from build123d import *

# Parameters (mm, degrees)
SKETCH2_W               = 1.1684
SKETCH2_H               = 0.7874
CUT_EXTRUDE1_DEPTH      = 3.7432
CUT_EXTRUDE1_DEPTH_BACK = 3.7432


with BuildPart() as part:
    # Sketch1 → Revolve1 (revolve)
    with BuildSketch(Plane.XY):
        with BuildLine():
            Line((0, 0), (0, 19.05))
            ThreePointArc((0, 19.05), (1.348059913, 18.449540529), (1.8034, 17.045801767))
            Line((1.8034, 17.045801767), (1.8034, 9.525))
            Line((1.8034, 9.525), (2.7432, 9.525))
            Line((2.7432, 9.525), (2.7432, 0))
            Line((2.7432, 0), (0, 0))
        make_face()
    revolve(axis=Axis((0, 0, 0), (0, 1, 0)))

    # Sketch2 → Cut-Extrude1 (cut, two sides)
    with BuildSketch(Plane.XY) as cut_extrude1_sk:
        with Locations((0, 0.3937)):
            Rectangle(SKETCH2_W, SKETCH2_H)
    extrude(amount=CUT_EXTRUDE1_DEPTH, mode=Mode.SUBTRACT)
    extrude(cut_extrude1_sk.sketch, amount=-CUT_EXTRUDE1_DEPTH_BACK, mode=Mode.SUBTRACT)


solid = part.part
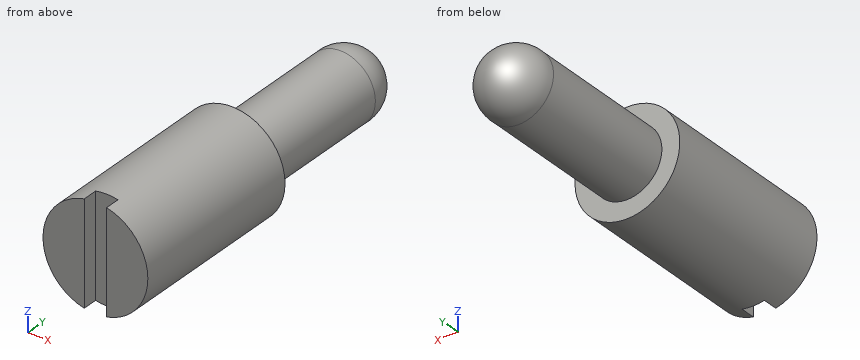
CAD build for the part. Positions are in the model's coordinates, mm. Give positions to 0.01 mm unless a question says otherwise; leave off trailing zeros. Order: outer loops, then holes, each group sorted by start corner. A loop starts at its lowest first (then second) coordinate and runs counter-clockwise, first axis right, second up. Notation, with made-up numbers: (4, 79) - (8, 79) arc R27 cw to (8, 106) - close; hole circle Ø1 at (58, 47.25). An arc over 180 degrees is marked (long way). Answer in a Markdown table with one row per item.
1. Saw through at B-B, the plane x = -1.3. Give the cut face in (y, z) (3 decimals).
Data:
| item | result |
|---|---|
| outline | (0, -2.416) - (9.525, -2.416) - (9.525, -1.25) - (17.046, -1.25) arc R1.264 ccw (long way) to (17.046, 1.25) - (9.525, 1.25) - (9.525, 2.416) - (0, 2.416) - close |
2. Probe probe 1 along Y at (x, z) = (1.2, -2.2) (3 decimals); probe 2 along X at (y, z) = (11, 0.05); probe 3 along Y at (x, z) = (0.3, 2.2) (3 decimals). List the from-to ranges inside material, lowest first. Write a range as [from, to].
Data:
| item | result |
|---|---|
| probe 1 | y = [0, 9.525] |
| probe 2 | x = [-1.8, 1.8] |
| probe 3 | y = [0.787, 9.525] |
3. Saw through at C-C, the plane y = 7.5. Give the cut face in (x, z).
Data:
| item | result |
|---|---|
| outline | circle Ø5.49 at (0, 0) |
4. Flat gauge pins, fed straight in: pin 1 (0.9 mm diameter, centred on y = 0.5, z = 1, fed in from +X); pin 2 (1 mm diameter, centred on x = 0.5, y = 17, fed in from +Z); pin 3 (1.5 mm diameter, centred on x = -1, y = 5.5, fed in from +Z). Where does each tip first touch, or does it go through?
Data:
| item | result |
|---|---|
| pin 1 | stops at x = 2.69 |
| pin 2 | stops at z = 1.81 |
| pin 3 | stops at z = 2.73 |
5. Saw through at D-D, the plane x = 0. Give the cut face in (y, z) (3 decimals), plus the area to 3 significant figures.
Data:
| item | result |
|---|---|
| outline | (0.787, -2.743) - (9.525, -2.743) - (9.525, -1.803) - (17.046, -1.803) arc R1.813 ccw (long way) to (17.046, 1.803) - (9.525, 1.803) - (9.525, 2.743) - (0.787, 2.743) - close |
| area | 80.9 mm² |
6. Saw through at A-A, the plane z = 0. Give the cut face in (x, y) (3 decimals), plus the area to 3 significant figures.
Data:
| item | result |
|---|---|
| outline | (-2.743, 0) - (-0.584, 0) - (-0.584, 0.787) - (0.584, 0.787) - (0.584, 0) - (2.743, 0) - (2.743, 9.525) - (1.803, 9.525) - (1.803, 17.046) arc R1.813 ccw (long way) to (-1.803, 17.046) - (-1.803, 9.525) - (-2.743, 9.525) - close |
| area | 84.3 mm² |
